The model under review builds one solid part; all positions refer to its coordinate system, in mm. A direction names the side the tool comes from. Round coordinates to 2 decimals unless told otherwise and drop trailing zeros. Order: outer loops, then holes, each group sorted by start corner. A loop starts at its lowest first (then second) coordinate and runs counter-clockwise, first axis right, second up.
from build123d import *

# Parameters (mm, degrees)
SKETCH1_W           = 900
SKETCH1_H           = 350
BOSS_EXTRUDE1_DEPTH = 15
CUT_EXTRUDE1_REACH  = 485.063
CUT_EXTRUDE2_REACH  = 485.063
SKETCH3_R           = 2
SKETCH10_R          = 2.75
CUT_EXTRUDE6_DEPTH  = 484.063142871
SKETCH11_R          = 1.75
CUT_EXTRUDE7_DEPTH  = 484.063142871
SKETCH12_R          = 2.75
CUT_EXTRUDE8_DEPTH  = 484.063142871
SKETCH13_R          = 2.5
CUT_EXTRUDE9_DEPTH  = 10
SKETCH14_R          = 2.5
CUT_EXTRUDE10_DEPTH = 10
SKETCH15_W          = 434.979135439
SKETCH15_H          = 130.036556738
CUT_EXTRUDE11_DEPTH = 484.063142871


with BuildPart() as part:
    # Sketch1 → Boss-Extrude1 (new body)
    with BuildSketch(Plane(origin=(0, 0, 0), x_dir=(1, 0, 0), z_dir=(0, 1, 0))):
        Rectangle(SKETCH1_W, SKETCH1_H)
    extrude(amount=BOSS_EXTRUDE1_DEPTH)

    # Sketch2 → Cut-Extrude1 (cut, up to next)
    with BuildSketch(Plane(origin=(0, 15, 0), x_dir=(1, 0, 0), z_dir=(0, 1, 0)), mode=Mode.PRIVATE) as cut_extrude1_sk1:
        with BuildLine():
            Line((-282.75, 23.5), (-282.75, 28.5))
            ThreePointArc((-282.75, 28.5), (-280, 31.25), (-277.25, 28.5))
            Line((-277.25, 28.5), (-277.25, 23.5))
            ThreePointArc((-277.25, 23.5), (-280, 20.75), (-282.75, 23.5))
        make_face()
    cut_extrude1_tool1 = extrude(cut_extrude1_sk1.sketch, amount=-CUT_EXTRUDE1_REACH, mode=Mode.PRIVATE) & part.part
    # Sketch2 → Cut-Extrude1 (cut, up to next)
    with BuildSketch(Plane(origin=(0, 15, 0), x_dir=(1, 0, 0), z_dir=(0, 1, 0)), mode=Mode.PRIVATE) as cut_extrude1_sk2:
        with BuildLine():
            Line((-327.25, 101.5), (-327.25, 96.5))
            ThreePointArc((-327.25, 96.5), (-330, 93.75), (-332.75, 96.5))
            Line((-332.75, 96.5), (-332.75, 101.5))
            ThreePointArc((-332.75, 101.5), (-330, 104.25), (-327.25, 101.5))
        make_face()
    cut_extrude1_tool2 = extrude(cut_extrude1_sk2.sketch, amount=-CUT_EXTRUDE1_REACH, mode=Mode.PRIVATE) & part.part
    # Sketch2 → Cut-Extrude1 (cut, up to next)
    with BuildSketch(Plane(origin=(0, 15, 0), x_dir=(1, 0, 0), z_dir=(0, 1, 0)), mode=Mode.PRIVATE) as cut_extrude1_sk3:
        with BuildLine():
            Line((-327.25, 28.5), (-327.25, 23.5))
            ThreePointArc((-327.25, 23.5), (-330, 20.75), (-332.75, 23.5))
            Line((-332.75, 23.5), (-332.75, 28.5))
            ThreePointArc((-332.75, 28.5), (-330, 31.25), (-327.25, 28.5))
        make_face()
    cut_extrude1_tool3 = extrude(cut_extrude1_sk3.sketch, amount=-CUT_EXTRUDE1_REACH, mode=Mode.PRIVATE) & part.part
    # Sketch2 → Cut-Extrude1 (cut, up to next)
    with BuildSketch(Plane(origin=(0, 15, 0), x_dir=(1, 0, 0), z_dir=(0, 1, 0)), mode=Mode.PRIVATE) as cut_extrude1_sk4:
        with BuildLine():
            Line((-282.75, 96.5), (-282.75, 101.5))
            ThreePointArc((-282.75, 101.5), (-280, 104.25), (-277.25, 101.5))
            Line((-277.25, 101.5), (-277.25, 96.5))
            ThreePointArc((-277.25, 96.5), (-280, 93.75), (-282.75, 96.5))
        make_face()
    cut_extrude1_tool4 = extrude(cut_extrude1_sk4.sketch, amount=-CUT_EXTRUDE1_REACH, mode=Mode.PRIVATE) & part.part
    add(cut_extrude1_tool1.solids().sort_by_distance((-280, 15, -26))[0], mode=Mode.SUBTRACT)
    add(cut_extrude1_tool2.solids().sort_by_distance((-330, 15, -99))[0], mode=Mode.SUBTRACT)
    add(cut_extrude1_tool3.solids().sort_by_distance((-330, 15, -26))[0], mode=Mode.SUBTRACT)
    add(cut_extrude1_tool4.solids().sort_by_distance((-280, 15, -99))[0], mode=Mode.SUBTRACT)

    # Sketch3 → Cut-Extrude2 (cut, up to next)
    with BuildSketch(Plane(origin=(0, 15, 0), x_dir=(1, 0, 0), z_dir=(0, 1, 0)), mode=Mode.PRIVATE) as cut_extrude2_sk1:
        with Locations(Location((-218.001464849, -53.5, 0), (0, 0, 270))):
            Circle(SKETCH3_R)
    cut_extrude2_tool1 = extrude(cut_extrude2_sk1.sketch, amount=-CUT_EXTRUDE2_REACH, mode=Mode.PRIVATE) & part.part
    # Sketch3 → Cut-Extrude2 (cut, up to next)
    with BuildSketch(Plane(origin=(0, 15, 0), x_dir=(1, 0, 0), z_dir=(0, 1, 0)), mode=Mode.PRIVATE) as cut_extrude2_sk2:
        with Locations(Location((-218.001464849, -150, 0), (0, 0, 270))):
            Circle(SKETCH3_R)
    cut_extrude2_tool2 = extrude(cut_extrude2_sk2.sketch, amount=-CUT_EXTRUDE2_REACH, mode=Mode.PRIVATE) & part.part
    # Sketch3 → Cut-Extrude2 (cut, up to next)
    with BuildSketch(Plane(origin=(0, 15, 0), x_dir=(1, 0, 0), z_dir=(0, 1, 0)), mode=Mode.PRIVATE) as cut_extrude2_sk3:
        with Locations(Location((-410, -150.75, 0), (0, 0, 270))):
            Circle(SKETCH3_R)
    cut_extrude2_tool3 = extrude(cut_extrude2_sk3.sketch, amount=-CUT_EXTRUDE2_REACH, mode=Mode.PRIVATE) & part.part
    add(cut_extrude2_tool1.solids().sort_by_distance((-218.001465, 15, 53.5))[0], mode=Mode.SUBTRACT)
    add(cut_extrude2_tool2.solids().sort_by_distance((-218.001465, 15, 150))[0], mode=Mode.SUBTRACT)
    add(cut_extrude2_tool3.solids().sort_by_distance((-410, 15, 150.75))[0], mode=Mode.SUBTRACT)

    # Sketch10 → Cut-Extrude6 (cut, through all)
    with BuildSketch(Plane(origin=(0, 15, 0), x_dir=(1, 0, 0), z_dir=(0, 1, 0))):
        with Locations(Location((-140, 38, 0), (0, 0, 270))):
            Circle(SKETCH10_R)
        with Locations(Location((-140, -2, 0), (0, 0, 270))):
            Circle(SKETCH10_R)
        with Locations(Location((-80, -2, 0), (0, 0, 270))):
            Circle(SKETCH10_R)
        with Locations(Location((-80, 38, 0), (0, 0, 270))):
            Circle(SKETCH10_R)
        with Locations(Location((-130, -32, 0), (0, 0, 270))):
            Circle(SKETCH10_R)
        with Locations(Location((-90, -32, 0), (0, 0, 270))):
            Circle(SKETCH10_R)
        with Locations(Location((-130, -72, 0), (0, 0, 270))):
            Circle(SKETCH10_R)
        with Locations(Location((-90, -72, 0), (0, 0, 270))):
            Circle(SKETCH10_R)
    extrude(amount=-CUT_EXTRUDE6_DEPTH, mode=Mode.SUBTRACT)

    # Sketch11 → Cut-Extrude7 (cut, through all)
    with BuildSketch(Plane(origin=(0, 15, 0), x_dir=(1, 0, 0), z_dir=(0, 1, 0))):
        with Locations(Location((-155, 88.5, 0), (0, 0, 270))):
            Circle(SKETCH11_R)
        with Locations(Location((-155, 41.5, 0), (0, 0, 270))):
            Circle(SKETCH11_R)
        with Locations(Location((-5, 88.5, 0), (0, 0, 270))):
            Circle(SKETCH11_R)
        with Locations(Location((-5, 41.5, 0), (0, 0, 270))):
            Circle(SKETCH11_R)
    extrude(amount=-CUT_EXTRUDE7_DEPTH, mode=Mode.SUBTRACT)

    # Sketch12 → Cut-Extrude8 (cut, through all)
    with BuildSketch(Plane(origin=(0, 15, 0), x_dir=(1, 0, 0), z_dir=(0, 1, 0))):
        with Locations(Location((272, 103, 0), (0, 0, 270))):
            Circle(SKETCH12_R)
        with Locations(Location((327, 103, 0), (0, 0, 270))):
            Circle(SKETCH12_R)
        with Locations(Location((272, 27, 0), (0, 0, 270))):
            Circle(SKETCH12_R)
        with Locations(Location((327, 27, 0), (0, 0, 270))):
            Circle(SKETCH12_R)
    extrude(amount=-CUT_EXTRUDE8_DEPTH, mode=Mode.SUBTRACT)

    # Sketch13 → Cut-Extrude9 (cut)
    with BuildSketch(Plane(origin=(0, 0, -175), x_dir=(-1, 0, 0), z_dir=(0, 0, -1))):
        with Locations((15, 7.5)):
            Circle(SKETCH13_R)
        with Locations((25, 7.5)):
            Circle(SKETCH13_R)
        with Locations((430, 7.5)):
            Circle(SKETCH13_R)
        with Locations((420, 7.5)):
            Circle(SKETCH13_R)
    cut_extrude9 = extrude(amount=-CUT_EXTRUDE9_DEPTH, mode=Mode.SUBTRACT)

    # Mirror1: Cut-Extrude9 across plane
    add(cut_extrude9.mirror(Plane.XY), mode=Mode.SUBTRACT)

    # Sketch14 → Cut-Extrude10 (cut)
    with BuildSketch(Plane.ZY.offset(450)):
        with Locations((-145, 7.5)):
            Circle(SKETCH14_R)
        with Locations((-135, 7.5)):
            Circle(SKETCH14_R)
        with Locations((145, 7.5)):
            Circle(SKETCH14_R)
        with Locations((135, 7.5)):
            Circle(SKETCH14_R)
    extrude(amount=-CUT_EXTRUDE10_DEPTH, mode=Mode.SUBTRACT)

    # Sketch15 → Cut-Extrude11 (cut, through all)
    with BuildSketch(Plane(origin=(0, 15, 0), x_dir=(1, 0, 0), z_dir=(0, 1, 0))):
        with Locations((232.51043228, -109.981721631)):
            Rectangle(SKETCH15_W, SKETCH15_H)
    extrude(amount=-CUT_EXTRUDE11_DEPTH, mode=Mode.SUBTRACT)


solid = part.part
(1) We need section C-C (y = 2.5). Count the separate pieces of the cut face and the enclosed holes in it, and give its area (3 significant figures).
(2) To check wall thickness, follow L1, parallel to X at y = 10.75, z = -27; L2, parallel to X at y = 9.5, z = 150; L3, parallel to X at y = 3, z = -41.5. State the ranges of each line that lie inside material, in increasing order.
(3) Clearance check with flat-ended pins moving along their axes: P1, Ø3, axis at x = -155, z = -88.5, coming from the +Y side; P2, Ø5.5, axis at x = -5, z = -41.5, coming from the -Y side; P3, Ø4.5, axis at x = -25, y = 7.5, coming from the +Z side; P4, Ø1, axis at x = 294.5, y = 9.5, coming from the +Z side. State where each tip first meets the part, or that it passes through.
(4) We need section A-A (z = 94). Give the boundary of the cut face in (x, y).
(5) Tool access review of faces 1 (the flat face through (-6, 7, -175)), 2 (the flat face through (229, 8, 44.963)): name each direction out of +Z, -Z, +X, -X, +Y, -Y from which nothing blocks a thin tool from reaching the whole face with its end or side.
(6) We need section B-B (x = 192.5). Give the boundary of the cut face in (y, z), and give its area (3 significant figures).
Verdict:
1. separate pieces: 1
1. enclosed holes: 23
1. area: 258,000 mm2
2. L1: x = -450 to -332.75, -327.25 to -282.75, -277.25 to 269.25, 274.75 to 324.25, 329.75 to 450
2. L2: x = -450 to -411.85, -408.15 to -220, -216 to 15.02
2. L3: x = -450 to -156.75, -153.25 to -6.75, -3.25 to 450
3. P1: passes through
3. P2: stops at y = 0
3. P3: stops at z = 165
3. P4: stops at z = 44.96
4. outline: (-450, 0) - (15.02, 0) - (15.02, 15) - (-450, 15) - close
5. face 1: -Z, +X, -X, +Y, -Y
5. face 2: +Z, +X, +Y, -Y
6. outline: (0, -175) - (15, -175) - (15, 44.96) - (0, 44.96) - close
6. area: 3,300 mm2
